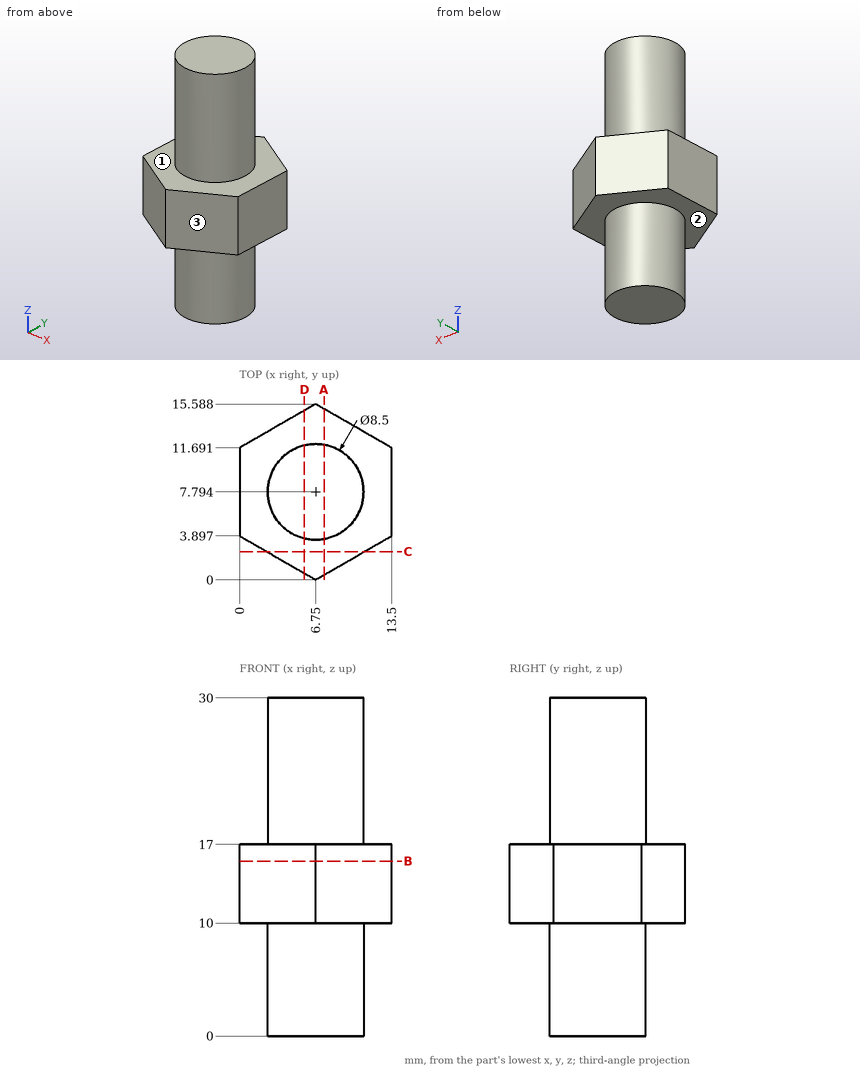
Design review of the part shown in the three views and the two pictorial views. Dimensions are in mm from the part's minimum x, y and z. A direction names the side the tool comes from. Give positions to 0.01 mm unless a question says otherwise; leave off trailing zeros. Write each loop counter-clockwise with the first axis right and the second up, starting at its lowest first coordinate (ties: lowest second). Pieces come first, ordered by that corner, then holes.
Item 1: Machinability: for the marked faces 1, 2 and 3, which of the approach directions +Z, -Z, +X, -X, +Y, -Y give a long, thin tool a straight path to every point of the face, cutting with its end or side? Answer none if there is none.
Item 2: Take a section at C-C (y = 2.5). Give the boundary of the cut face in (x, z).
Item 3: Take a section at B-B (z = 15.5). Give the boundary of the cut face in (x, y), and give its area (3 significant figures).
Item 4: Wall thickness on probe 1 along Z at (x, y) = (1, 12); probe 2 along Y at (x, z) = (6.5, 28.5); probe 3 along X at (y, z) = (3.5, 13.25) (1 decimal): over which ranges is each line inside the solid? List them lowest first.
Item 5: Take a section at D-D (x = 5.75). Give the boundary of the cut face in (y, z) (1 decimal).
Item 6: Insertion check: P1, Ø5, axis at x = 9.5, z = 17, coming from the +Y side (1 decimal); P2, Ø2, axis at x = 7.5, z = 7.5, coming from the +Y side; P3, Ø5, axis at y = 12, z = 5, coming from the -X side. Each pin has a flat end and moves straight along its axis. Give the tip position at first contact, or say it passes through.
Item 7: Take a section at A-A (x = 7.5). Give the boundary of the cut face in (y, z) (1 decimal).
Established:
1. face 1: +Z
1. face 2: -Z
1. face 3: +Z, -Z, +X, -Y
2. outline: (2.42, 10) - (11.08, 10) - (11.08, 17) - (2.42, 17) - close
3. outline: (0, 3.9) - (6.75, 0) - (13.5, 3.9) - (13.5, 11.69) - (6.75, 15.59) - (0, 11.69) - close
3. area: 158 mm2
4. probe 1: z = 10 to 17
4. probe 2: y = 3.55 to 12.04
4. probe 3: x = 0.7 to 12.8
5. outline: (0.6, 10) - (3.7, 10) - (3.7, 0) - (11.9, 0) - (11.9, 10) - (15, 10) - (15, 17) - (11.9, 17) - (11.9, 30) - (3.7, 30) - (3.7, 17) - (0.6, 17) - close
6. P1: stops at y = 15.4
6. P2: stops at y = 12.04
6. P3: stops at x = 2.86
7. outline: (0.4, 10) - (3.6, 10) - (3.6, 0) - (12, 0) - (12, 10) - (15.2, 10) - (15.2, 17) - (12, 17) - (12, 30) - (3.6, 30) - (3.6, 17) - (0.4, 17) - close
